Can you work these out from the model? Positions are in its coordinate system, mm. A direction names the side the tool comes from. Coordinates: 2 decimals unless noted, no trailing zeros. Order: outer loops, then holes, each group sorted by start corner. A loop starts at its lowest first (then second) coordinate and runs counter-clockwise, first axis right, second up. Notation, with made-up numbers: (23, 20) -> (33, 20) arc R12 ccw to (33, 26) -> close; hole circle Ø2 at (5.25, -20). An arc over 180 degrees is marked (long way). Answer in a Markdown table with one row per item.
```python
from build123d import *

# Parameters (mm, degrees)
PAD_DEPTH    = 6.5
SKETCH001_R  = 2
POCKET_DEPTH = 34.999843
FILLET_R     = 2
FILLET001_R  = 2
FILLET002_R  = 6
FILLET003_R  = 2
FILLET004_R  = 2
FILLET005_R  = 2


with BuildPart() as part:
    # Sketch → Pad (new body, symmetric)
    with BuildSketch(Plane.XY):
        Polygon((-8.5, 9.102282), (-8.5, -9.297718), (8.5, -9.297718), (8.5, 9.102282), (26.498843, 9.102282), (26.498843, 59.102282), (18.498843, 59.102282), (18.498843, 19.102282), (-18.498843, 19.102282), (-18.498843, 59.102282), (-26.498843, 59.102282), (-26.498843, 9.102282), align=None)
    extrude(amount=PAD_DEPTH, both=True)

    # Sketch001 → Pocket (cut, through all)
    with BuildSketch(Plane.YZ.offset(8.5)):
        with Locations((-2.397718, 0)):
            Circle(SKETCH001_R)
    extrude(amount=-POCKET_DEPTH, mode=Mode.SUBTRACT)

    # Fillet
    fillet_edges = [part.edges().sort_by_distance(p)[0] for p in [
        (-18.498843, 19.102282, 0),
    ]]
    fillet(fillet_edges, radius=FILLET_R)

    # Fillet001
    fillet001_edges = [part.edges().sort_by_distance(p)[0] for p in [
        (18.498843, 19.102282, 0),
    ]]
    fillet(fillet001_edges, radius=FILLET001_R)

    # Fillet002
    fillet002_edges = [part.edges().sort_by_distance(p)[0] for p in [
        (26.498843, 9.102282, 0),
        (-26.498843, 9.102282, 0),
    ]]
    fillet(fillet002_edges, radius=FILLET002_R)

    # Fillet003
    fillet003_edges = [part.edges().sort_by_distance(p)[0] for p in [
        (-24.741484, 10.859642, 6.5),
        (-26.498843, 37.102282, 6.5),
        (-14.499422, 9.102282, 6.5),
        (-14.499422, 9.102282, -6.5),
        (-24.741484, 10.859642, -6.5),
        (-26.498843, 37.102282, -6.5),
    ]]
    fillet(fillet003_edges, radius=FILLET003_R)

    # Fillet004
    fillet004_edges = [part.edges().sort_by_distance(p)[0] for p in [
        (14.499422, 9.102282, 6.5),
        (24.741484, 10.859642, 6.5),
        (26.498843, 37.102282, 6.5),
        (26.498843, 37.102282, -6.5),
        (24.741484, 10.859642, -6.5),
        (14.499422, 9.102282, -6.5),
    ]]
    fillet(fillet004_edges, radius=FILLET004_R)

    # Fillet005
    fillet005_edges = [part.edges().sort_by_distance(p)[0] for p in [
        (18.498843, 59.102282, 0),
        (-18.498843, 59.102282, 0),
    ]]
    fillet(fillet005_edges, radius=FILLET005_R)


solid = part.part
```
(1) Suppose I cut it at C-C (x = 15). Please give me the cut outline in (y, z).
Response values:
| item | result |
|---|---|
| outline | (9.1, -4.5) arc R2 ccw to (11.1, -6.5) -> (19.1, -6.5) -> (19.1, 6.5) -> (11.1, 6.5) arc R2 ccw to (9.1, 4.5) -> close |
(2) Will these pins go through, and if not, where does the flat tip stop? pin 1 Ø5 at (y, z) = (-2.4, 0) entering from +X; pin 2 Ø1 at (x, z) = (-9.5, 5) entering from +Y; pin 3 Ø4.5 at (x, z) = (17.5, -0.5) entering from -Y.
Response values:
| item | result |
|---|---|
| pin 1 | x = 8.5 |
| pin 2 | y = 19.1 |
| pin 3 | y = 9.1 |
(3) On a 3-axis mill with a long thin cutter (end or side, diameter ignored), from which of +Z, -Z, +X, -X, +Y, -Y can I reach the whole of each face in a straight line? I mean faces 1 (the cylindrical face through (-14.415, 9.673, 5.899)), 2 (the cylindrical face through (14.583, 9.704, -5.93)), 3 (the flat face through (-15, 9.102, 0)), 4 (the flat face through (0, 19.102, 0)), 5 (the cylindrical face through (-14.415, 9.704, -5.93)). Say none if no direction works.
Response values:
| item | result |
|---|---|
| face 1 | +Z, -X, -Y |
| face 2 | -Z, +X, -Y |
| face 3 | +Z, -Z, -X, -Y |
| face 4 | +Z, -Z, +Y |
| face 5 | -Z, -X, -Y |
(4) Suppose I cut it at D-D (x = -7.5). Please give me the cut outline in (y, z).
Response values:
| item | result |
|---|---|
| outline | (-9.3, -6.5) -> (19.1, -6.5) -> (19.1, 6.5) -> (-9.3, 6.5) -> close; hole circle Ø4 at (-2.4, 0) |
(5) Suppose I cut it at A-A (y = 28.5). Please give me the cut outline in (x, z).
Response values:
| item | result |
|---|---|
| outline | (-26.5, -4.5) arc R2 ccw to (-24.5, -6.5) -> (-18.5, -6.5) -> (-18.5, 6.5) -> (-24.5, 6.5) arc R2 ccw to (-26.5, 4.5) -> close; (18.5, -6.5) -> (24.5, -6.5) arc R2 ccw to (26.5, -4.5) -> (26.5, 4.5) arc R2 ccw to (24.5, 6.5) -> (18.5, 6.5) -> close |
(6) I need wall thicknesses on line 1 (X direction, y = 39, z = -1.75); line 2 (Y direction, x = 13, z = -2.75); line 3 (X direction, y = 49.5, z = -5.25). Which ranges of each line are inside material? Lowest first, please. Write a range as [from, to].
Response values:
| item | result |
|---|---|
| line 1 | [-26.5, -18.5], [18.5, 26.5] |
| line 2 | [9.1, 19.1] |
| line 3 | [-26.35, -18.5], [18.5, 26.35] |
(7) Suppose I cut it at B-B (z = 0). Please give me the cut outline in (x, y), and give its area (3 significant figures).
Response values:
| item | result |
|---|---|
| outline | (-26.5, 15.1) arc R6 ccw to (-20.5, 9.1) -> (-8.5, 9.1) -> (-8.5, -0.4) -> (8.5, -0.4) -> (8.5, 9.1) -> (20.5, 9.1) arc R6 ccw to (26.5, 15.1) -> (26.5, 59.1) -> (20.5, 59.1) arc R2 ccw to (18.5, 57.1) -> (18.5, 21.1) arc R2 cw to (16.5, 19.1) -> (-16.5, 19.1) arc R2 cw to (-18.5, 21.1) -> (-18.5, 57.1) arc R2 ccw to (-20.5, 59.1) -> (-26.5, 59.1) -> close; (-8.5, -9.3) -> (8.5, -9.3) -> (8.5, -4.4) -> (-8.5, -4.4) -> close |
| area | 1,400 mm2 |
(8) We'd pull the mould along X, two halves only. Please class faces 6 (the flat face through (-8.5, 1, 0)), 7 (the flat face through (-23, 59.102, 0)), 8 (the flat face through (-18.499, 39, 0)): +X half, -X half, draft (parallel to the pull), parting line (faces both ways), or undercut.
Response values:
| item | result |
|---|---|
| face 6 | -X half |
| face 7 | draft |
| face 8 | undercut |
